Read the model definition and answer for the solid it produces. Units are mm, in the model's axes. Face numbers are marked on the shaded views. A direction names the side the tool comes from. Give positions to 0.01 mm unless a question says otherwise; leave off trailing zeros. Loops run counter-clockwise (first coordinate to the right, second up) from the corner with the lowest first, then second, coordinate; pieces in that order, holes last.
(1) Which of the six approach directions +Z, -Z, +X, -X, +Y, -Y give full straight-line access (tool end or side, diameter ignored) to the marked faces 5, 6 and 7?
(2) Find section A-A, the plane z = -4. Write down the section's boundary in (x, y).
(3) Find section C-C, the plane y = -8.5. Write down the section's boundary in (x, z).
(4) Find section B-B, the plane x = -3.25. Write down the section's boundary in (y, z).
(5) Find section D-D, the plane z = 4. Write down the section's boundary in (x, y).
(6) Straight lines are drawn through the part: probe 1 along X at (y, z) = (-6.75, 16); probe 2 along X at (y, z) = (0.15, -4); probe 3 along Z at (x, y) = (0, 6.9). For each, find the intervals that lie inside material, in ascending order.
(7) Each of these flat-tipped pins is pushed along its axis until it touches: P1, Ø2, axis at x = -0.5, z = 7.5, coming from the -Y side; P2, Ø1.3, axis at y = -1.5, z = 12, coming from the +X side; P3, Ø8, axis at y = 1.5, z = 5.5, coming from the +X side; P4, Ø1.8, axis at x = 0, z = -4, coming from the -Y side. Where does it stop, or does it pass through?
(8) Determine the mould class of the marked faces 1, 2, 3 and 4 for opening direction Y: pulls with the +Y half, pulls with the -Y half, needs draft (parallel to the pull), parting line crosses it, or undercut.
Autodesk Fusion 360 part; units mm, degrees
sketch "Sketch1" plane through (0, 0, 0) normal (0, 0, 1) x (1, 0, 0)
  line L0 (6.25, 9.25) -> (-6.25, 9.25)
  line L1 (-6.25, 9.25) -> (-6.25, -9.25)
  line L2 (-6.25, -9.25) -> (6.25, -9.25)
  line L3 (6.25, -9.25) -> (6.25, 9.25)
  line L4 (6.25, 9.25) -> (-6.25, -9.25) construction
  line L5 (-6.25, 9.25) -> (6.25, -9.25) construction
  dimension "d1" = 12.5
  dimension "d2" = 18.5
extrude "Extrude1" add sketch "Sketch1" along normal blind 10 makes body 1
sketch "Sketch2" plane through (0, 0, 10) normal (0, 0, 1) x (-1, 0, 0)
  line L0 (-6.25, 9.25) -> (-6.25, -9.25)
  line L1 (-6.25, -9.25) -> (6.25, -9.25)
  line L2 (6.25, -9.25) -> (6.25, 9.25)
  line L3 (6.25, 9.25) -> (-6.25, 9.25)
  line L4 (-6.5, -10) -> (6.5, -10)
  line L5 (6.5, -10) -> (6.5, 10)
  line L6 (6.5, 10) -> (-6.5, 10)
  line L7 (-6.5, 10) -> (-6.5, -10)
  line L8 (-6.5, -10) -> (6.5, 10) construction
  line L9 (6.5, -10) -> (-6.5, 10) construction
  dimension "d5" = 13
  dimension "d6" = 20
extrude "Extrude2" add sketch "Sketch2" along normal blind 4.5 contours L0 L1 L2 L3 | L4 L5 L6 L7 bodies 1
sketch "Sketch3" plane through (0, 0, 14.5) normal (0, 0, 1) x (-1, 0, 0)
  line L0 (-6.5, 10) -> (-6.5, -10)
  line L1 (-6.5, -10) -> (6.5, -10)
  line L2 (6.5, -10) -> (6.5, 10)
  line L3 (6.5, 10) -> (-6.5, 10)
  line L4 (-7.5, -10.5) -> (7.5, -10.5)
  line L5 (7.5, -10.5) -> (7.5, 10.5)
  line L6 (7.5, 10.5) -> (-7.5, 10.5)
  line L7 (-7.5, 10.5) -> (-7.5, -10.5)
  line L8 (-7.5, -10.5) -> (7.5, 10.5) construction
  line L9 (7.5, -10.5) -> (-7.5, 10.5) construction
  dimension "d9" = 15
  dimension "d10" = 21
extrude "Extrude3" add sketch "Sketch3" along normal blind 2 contours L0 L1 L2 L3 | L4 L5 L6 L7 bodies 1
sketch "Sketch4" plane through (0, 0, 16.5) normal (0, 0, 1) x (-1, 0, 0)
  line L0 (-7.5, 10.5) -> (-7.5, -10.5)
  line L1 (-7.5, -10.5) -> (7.5, -10.5)
  line L2 (7.5, -10.5) -> (7.5, 10.5)
  line L3 (7.5, 10.5) -> (-7.5, 10.5)
  line L4 (-5, -7.5) -> (5, -7.5)
  line L5 (5, -7.5) -> (5, 7.5)
  line L6 (5, 7.5) -> (-5, 7.5)
  line L7 (-5, 7.5) -> (-5, -7.5)
  line L8 (-5, -7.5) -> (5, 7.5) construction
  line L9 (5, -7.5) -> (-5, 7.5) construction
  dimension "d13" = 10
  dimension "d14" = 15
extrude "Extrude4" add sketch "Sketch4" along normal blind 3.5 contours L4 L5 L6 L7 bodies 1
sketch "Sketch5" plane through (5, 0, 0) normal (1, 0, 0) x (0, 1, 0)
  line L0 (-7.5, 16.5) -> (7.5, 16.5)
  line L1 (7.5, 16.5) -> (7.5, 20)
  line L2 (7.5, 20) -> (-7.5, 20)
  line L3 (-7.5, 20) -> (-7.5, 16.5)
  line L4 (0, 16.5) -> (7.5, 16.5)
  line L5 (0, 16.5) -> (-6.6332, 20)
  line L6 (-6.6332, 20) -> (-7.5, 16.5)
  dimension "d17" = 7.5
extrude "Extrude5" cut sketch "Sketch5" against normal blind 10 contours L2 L3 L6 | L0 L1 L2 L4 L5 bodies 1
sketch "Sketch6" plane through (0, 0, 16.5) normal (0, 0, 1) x (-1, 0, 0)
  line L0 (-5, 7.5) -> (5, 7.5)
  line L1 (5, 7.5) -> (5, 0)
  line L2 (5, 0) -> (-5, 0)
  line L3 (-5, 0) -> (-5, 7.5)
  line L4 (-7.5, 10.5) -> (-7.5, -10.5)
  line L5 (-7.5, -10.5) -> (7.5, -10.5)
  line L6 (7.5, -10.5) -> (7.5, 10.5)
  line L7 (7.5, 10.5) -> (-7.5, 10.5)
  line L8 (-5, -7.5) -> (5, -7.5)
  line L9 (5, -7.5) -> (5, 7.5)
  line L10 (5, 7.5) -> (-5, 7.5)
  line L11 (-5, 7.5) -> (-5, -7.5)
  line L12 (-5, -7.5) -> (5, 7.5) construction
  line L13 (5, -7.5) -> (-5, 7.5) construction
  line L14 (5.5, 8) -> (-5.5, 8)
  line L15 (-5.5, 8) -> (-5.5, -8)
  line L16 (-5.5, -8) -> (5.5, -8)
  line L17 (5.5, -8) -> (5.5, 8)
  dimension "d20" = 10
  dimension "d21" = 15
  dimension "d22" = 0.5
extrude "Extrude6" cut sketch "Sketch6" against normal blind 4 contours L14 L15 L16 L17 bodies 1
fillet "Fillet1" radius 1.5 4 edges at (7.5, -10.5, 15.5) (-7.5, -10.5, 15.5) (-7.5, 10.5, 15.5) (7.5, 10.5, 15.5) on bodies 1
fillet "Fillet2" radius 0.5 8 edges at (-7.0607, 10.0607, 16.5) (-7.5, 0, 16.5) (-7.0607, -10.0607, 16.5) (0, -10.5, 16.5) (7.0607, -10.0607, 16.5) (7.5, 0, 16.5) (7.0607, 10.0607, 16.5) (0, 10.5, 16.5) on bodies 1
fillet "Fillet3" radius 10 1 edges at (0, 0, 16.5) on bodies 1
fillet "Fillet4" radius 0.5 2 edges at (0, 7.5, 16.5) (0, -6.6332, 20) on bodies 1
fillet "Fillet5" radius 0.5 14 edges at (-5, -7.1434, 17.9399) (-5, -6.506, 19.7159) (-5, -4.1292, 18.6788) (-5, 0.0726, 16.7932) (-5, 4.7382, 16.5) (-5, 7.3536, 16.3536) (-5, 7.5, 14.25) (5, 7.5, 14.25) (5, 7.3536, 16.3536) (5, 4.7382, 16.5) (5, 0.0726, 16.7932) (5, -4.1292, 18.6788) (5, -6.506, 19.7159) (5, -7.1434, 17.9399) on bodies 1
sketch "Sketch7" plane through (0, 0, 16.5) normal (0, 0, 1) x (-1, 0, 0)
  line L0 (-4.5, -2.4764) -> (-4.5, -7)
  line L1 (-4.5, -7) -> (4.5, -7)
  line L2 (4.5, -7) -> (4.5, -2.4764)
  line L3 (4.5, -2.4764) -> (-4.5, -2.4764)
  line L4 (-4.5, -7) -> (4.5, -2.4764) construction
  circle A0 centre (0, -4.7382) radius 1.5
  dimension "d35" = 3
extrude "Extrude7" add sketch "Sketch7" along normal blind 0.5 draft -45 contours A0 bodies 1
fillet "Fillet6" radius 0.5 1 edges at (0.9323, 4.3766, 17) on bodies 1
sketch "Sketch8" plane through (0, 0, 0) normal (0, 0, -1) x (1, 0, 0)
  line L0 (6.25, -9.25) -> (6.25, 9.25)
  line L1 (6.25, 9.25) -> (-6.25, 9.25)
  line L2 (-6.25, 9.25) -> (-6.25, -9.25)
  line L3 (-6.25, -9.25) -> (6.25, -9.25)
  line L4 (2.5, 7.5) -> (-2.5, 7.5) construction
  line L5 (-2.5, 7.5) -> (-2.5, -7.5) construction
  line L6 (-2.5, -7.5) -> (2.5, -7.5) construction
  line L7 (2.5, -7.5) -> (2.5, 7.5) construction
  line L8 (2.5, 7.5) -> (-2.5, -7.5) construction
  line L9 (-2.5, 7.5) -> (2.5, -7.5) construction
  line L10 (-2.5, 7.5) -> (2.5, 7.5)
  line L11 (2.5, 7.5) -> (2.5, 6.5)
  line L12 (2.5, 6.5) -> (-2.5, 6.5)
  line L13 (-2.5, 6.5) -> (-2.5, 7.5)
  line L14 (-2.5, -7.5) -> (2.5, -7.5)
  line L15 (2.5, -7.5) -> (2.5, -6.5)
  line L16 (2.5, -6.5) -> (-2.5, -6.5)
  line L17 (-2.5, -6.5) -> (-2.5, -7.5)
  line L18 (2.5, 0.5) -> (-2.5, 0.5)
  line L19 (-2.5, 0.5) -> (-2.5, -0.5)
  line L20 (-2.5, -0.5) -> (2.5, -0.5)
  line L21 (2.5, -0.5) -> (2.5, 0.5)
  line L22 (2.5, 0.5) -> (-2.5, -0.5) construction
  line L23 (-2.5, 0.5) -> (2.5, -0.5) construction
  dimension "d40" = 5
  dimension "d41" = 15
  dimension "d42" = 5
  dimension "d43" = 1
  dimension "d44" = 5
  dimension "d45" = 1
  dimension "d46" = 5
  dimension "d47" = 1
extrude "Extrude8" add sketch "Sketch8" along normal blind 7 separate body contours L10 L11 L12 L13 | L14 L15 L16 L17 | L18 L19 L20 L21 makes body 2 at (0.8333, 6.5, -2.3333) makes body 3 at (-0.8333, 0.5, -2.3333) makes body 4 at (-0.8333, -7.5, -2.3333)
sketch "Sketch9" plane through (0, 7.5, 0) normal (0, 1, 0) x (-1, 0, 0)
  line L0 (2.5, 0) -> (-2.5, 0)
  line L1 (-2.5, 0) -> (-2.5, -7)
  line L2 (-2.5, -7) -> (2.5, -7)
  line L3 (2.5, -7) -> (2.5, 0)
  line L4 (0, -7) -> (0, -4)
  circle A0 centre (0, -4) radius 1
  dimension "d50" = 3
  dimension "d51" = 2
extrude "Extrude9" cut sketch "Sketch9" against normal blind 15 contours A0 bodies 2 3 4
chamfer "Chamfer1" distance 1 angle 45 6 edges at (2.5, -7, -7) (-2.5, -7, -7) (2.5, 0, -7) (-2.5, 0, -7) (2.5, 7, -7) (-2.5, 7, -7) on bodies 2 3 4
combine "Combine1" operation add target body 1 tool bodies 2 3 4
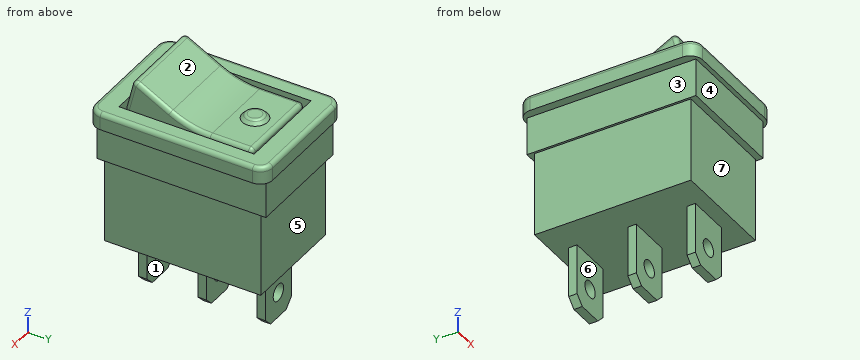
Entries:
1. face 5: -Z, +X, -X, +Y
1. face 6: -Z, +X, -X
1. face 7: -Z, +X, -X, -Y
2. outline: (-2.5, -7.5) - (-1, -7.5) - (-1, -6.5) - (-2.5, -6.5) - close; (-2.5, -0.5) - (-1, -0.5) - (-1, 0.5) - (-2.5, 0.5) - close; (-2.5, 6.5) - (-1, 6.5) - (-1, 7.5) - (-2.5, 7.5) - close; (1, -7.5) - (2.5, -7.5) - (2.5, -6.5) - (1, -6.5) - close; (1, -0.5) - (2.5, -0.5) - (2.5, 0.5) - (1, 0.5) - close; (1, 6.5) - (2.5, 6.5) - (2.5, 7.5) - (1, 7.5) - close
3. outline: (-7.5, 14.5) - (-6.5, 14.5) - (-6.5, 10) - (-6.25, 10) - (-6.25, 0) - (6.25, 0) - (6.25, 10) - (6.5, 10) - (6.5, 14.5) - (7.5, 14.5) - (7.5, 16) arc R0.5 ccw to (7, 16.5) - (-7, 16.5) arc R0.5 ccw to (-7.5, 16) - close
4. outline: (-10.5, 14.5) - (-10, 14.5) - (-10, 10) - (-9.25, 10) - (-9.25, 0) - (9.25, 0) - (9.25, 10) - (10, 10) - (10, 14.5) - (10.5, 14.5) - (10.5, 16) arc R0.5 ccw to (10, 16.5) - (8, 16.5) - (8, 12.5) - (7.5, 12.5) - (7.5, 16) arc R0.5 ccw to (7, 16.5) - (2.48, 16.5) arc R10 cw to (-2.19, 17.66) - (-6.07, 19.7) arc R0.5 ccw to (-6.79, 19.38) - (-7.5, 16.5) - (-7.5, 12.5) - (-8, 12.5) - (-8, 16.5) - (-10, 16.5) arc R0.5 ccw to (-10.5, 16) - close
5. outline: (-6.25, -9.25) - (6.25, -9.25) - (6.25, 9.25) - (-6.25, 9.25) - close
6. probe 1: x = -7.5 to -5.5, -5 to 5, 5.5 to 7.5
6. probe 2: x = -2.5 to -1, 1 to 2.5
6. probe 3: z = -7 to -5, -3 to 16.5
7. P1: stops at y = -9.25
7. P2: stops at x = 6.5
7. P3: stops at x = 6.25
7. P4: passes through
8. face 1: undercut
8. face 2: pulls with the +Y half
8. face 3: needs draft
8. face 4: pulls with the -Y half
